Geometry check sheet. Reference: the model listing, model coordinates, mm. Coordinates: 2 decimals unless noted, no trailing zeros. Write each loop counter-clockwise with the first axis right and the second up, starting at its lowest first coordinate (ties: lowest second). Pieces come first, ordered by that corner, then holes. Notation, with made-up numbers: (-15, 51.5) - (30, 51.5) arc R12 cw to (30, 74.5) - close; hole circle Ø5 at (-20.5, -38.75). An arc over 180 degrees is marked (long way). Answer as a JSON object with one key per item and string values. Group by question number.
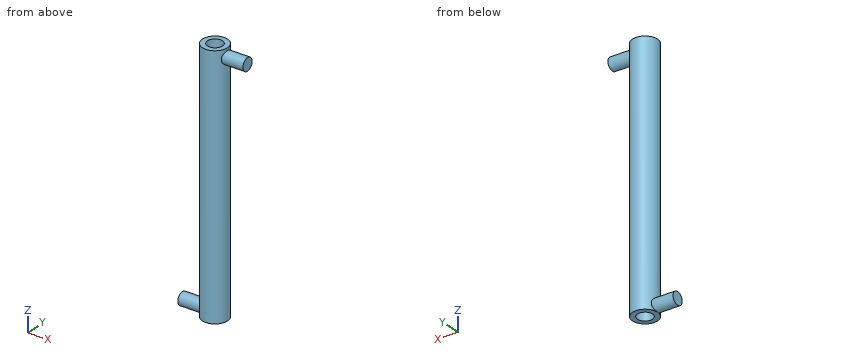
from build123d import *

# Parameters (mm, degrees)
F0_R     = 50
F0_R_2   = 30
F1_DEPTH = 1000
F3_R     = 25
F4_DEPTH = 100
F6_R     = 25
F7_DEPTH = 100


with BuildPart() as f1:
    # F0 (on Top) → F1 (new body)
    with BuildSketch(Plane.XY):
        Circle(F0_R)
        Circle(F0_R_2, mode=Mode.SUBTRACT)
    extrude(amount=F1_DEPTH)

    # F3 (on offset) → F4 (join)
    with BuildSketch(Plane.YZ.offset(-130)):
        with Locations((0, 25.231782)):
            Circle(F3_R)
    extrude(amount=F4_DEPTH)

    # F6 (on offset) → F7 (join)
    with BuildSketch(Plane.YZ.offset(130)):
        with Locations((0, 964.894772)):
            Circle(F6_R)
    extrude(amount=-F7_DEPTH)


solid = f1.part
(1) Material ranges on L1, parallel to Y at x = 0, z = 718; L2, parallel to Y at x = -19, z = 519.5; L3, parallel to X at y = -19.5, z = 447, recorded low to high. Write a range as [from, to].
(2) Section check C-C (z = 572). Record the cut outline in (x, y).
(3) Gauge pin test, flat ends, axial feed: pin 1 (5 mm diameter, centred on y = 8.5, z = 631.5, fed in from -X); pin 2 (6 mm diameter, centred on x = -21.5, z = 266.5, fed in from +Y); pin 3 (4 mm diameter, centred on y = 11, z = 206.5, fed in from +X). Record the tip position at first contact, or that the pin passes through.
(4) Section check D-D (y = 38.5). Record the cut outline in (x, z).
(5) Section check A-A (x = 0). Record the cut outline in (y, z).
(6) Section check B-B (y = 0). Record the cut outline in (x, z), and give its area (3 significant figures).
Conclusion:
{
 "1": {"L1": "y = [-50, -30], [30, 50]", "L2": "y = [-46.25, -23.22], [23.22, 46.25]", "L3": "x = [-46.04, -22.8], [22.8, 46.04]"},
 "2": {"outline": "circle Ø100 at (0, 0); hole circle Ø60 at (0, 0)"},
 "3": {"pin 1": "stops at x = -49.64", "pin 2": "stops at y = 46.45", "pin 3": "stops at x = 49.18"},
 "4": {"outline": "(-31.9, 0) - (31.9, 0) - (31.9, 1000) - (-31.9, 1000) - close"},
 "5": {"outline": "(-50, 0) - (-30, 0) - (-30, 1000) - (-50, 1000) - close; (30, 0) - (50, 0) - (50, 1000) - (30, 1000) - close"},
 "6": {"outline": "(-130, 0.23) - (-50, 0.23) - (-50, 0) - (-30, 0) - (-30, 1000) - (-50, 1000) - (-50, 50.23) - (-130, 50.23) - close; (30, 0) - (50, 0) - (50, 939.89) - (130, 939.89) - (130, 989.89) - (50, 989.89) - (50, 1000) - (30, 1000) - close", "area": "48,000 mm^2"}
}
